from build123d import *

# Parameters (mm, degrees)
BOSS_EXTRUDE1_DEPTH = 8
SKETCH2_R           = 3.8805
CUT_EXTRUDE1_DEPTH  = 10
SKETCH5_W           = 15
SKETCH5_H           = 85
SKETCH5_R           = 2.5
SKETCH5_W_2         = 25
SKETCH5_H_2         = 105
SKETCH5_W_3         = 30
CUT_EXTRUDE4_DEPTH  = 1
CUT_EXTRUDE7_START  = 91
SKETCH10_R          = 2.5
CUT_EXTRUDE7_DEPTH  = 91
SKETCH12_W          = 165
SKETCH12_H          = 10
SKETCH12_R          = 2
CUT_EXTRUDE11_DEPTH = 3
SKETCH14_R          = 2.5
CUT_EXTRUDE14_DEPTH = 22


with BuildPart() as part:
    # Sketch1 → Boss-Extrude1 (new body)
    with BuildSketch(Plane.XY):
        Polygon((307.812229203, 127.5), (127.5, 307.812229203), (-127.5, 307.812229203), (-307.812229203, 127.5), (-307.812229203, -127.5), (-127.5, -307.812229203), (127.5, -307.812229203), (307.812229203, -127.5), align=None)
    extrude(amount=BOSS_EXTRUDE1_DEPTH)

    # Sketch2 → Cut-Extrude1 (cut)
    with BuildSketch(Plane.XY.offset(8)):
        with Locations((0, 200)):
            Circle(SKETCH2_R)
        with Locations((0, -200)):
            Circle(SKETCH2_R)
        Polygon((212.5, 105), (212.5, -105), (267.5, -105), (267.5, -40), (268.5, -40), (268.5, 0), (268.5, 40), (267.5, 40), (267.5, 105), align=None)
        Polygon((-267.5, 105), (-212.5, 105), (-212.5, -105), (-267.5, -105), (-267.5, -40), (-268.5, -40), (-268.5, 0), (-268.5, 40), (-267.5, 40), align=None)
    extrude(amount=-CUT_EXTRUDE1_DEPTH, mode=Mode.SUBTRACT)

    # Sketch5 → Cut-Extrude4 (cut)
    # profile 1 of 6: a face of its own
    with BuildSketch(Plane.XY.offset(8)):
        with Locations((80.5, 2.5)):
            Rectangle(SKETCH5_W, SKETCH5_H)
        with Locations(Location((78, 32.5, 0), (0, 0, 180))):
            Circle(SKETCH5_R, mode=Mode.SUBTRACT)
        with Locations(Location((78, -32.5, 0), (0, 0, 180))):
            Circle(SKETCH5_R, mode=Mode.SUBTRACT)
    # profile 2 of 6: a face of its own
    with BuildSketch(Plane.XY.offset(8)):
        with Locations((-185.5, 2.5)):
            Rectangle(SKETCH5_W_2, SKETCH5_H_2)
        with Locations((-183, -40)):
            Circle(SKETCH5_R, mode=Mode.SUBTRACT)
        with Locations((-183, 40)):
            Circle(SKETCH5_R, mode=Mode.SUBTRACT)
    # profile 3 of 6: a face of its own
    with BuildSketch(Plane.XY.offset(8)):
        with Locations((-133, 2.5)):
            Rectangle(SKETCH5_W_3, SKETCH5_H_2)
        with Locations((-133, -40)):
            Circle(SKETCH5_R, mode=Mode.SUBTRACT)
        with Locations((-133, 40)):
            Circle(SKETCH5_R, mode=Mode.SUBTRACT)
    # profile 4 of 6: a face of its own
    with BuildSketch(Plane.XY.offset(8)):
        with Locations((-80.5, 2.5)):
            Rectangle(SKETCH5_W, SKETCH5_H)
        with Locations((-78, -32.5)):
            Circle(SKETCH5_R, mode=Mode.SUBTRACT)
        with Locations((-78, 32.5)):
            Circle(SKETCH5_R, mode=Mode.SUBTRACT)
    # profile 5 of 6: a face of its own
    with BuildSketch(Plane.XY.offset(8)):
        with Locations((133, 2.5)):
            Rectangle(SKETCH5_W_3, SKETCH5_H_2)
        with Locations(Location((133, 40, 0), (0, 0, 180))):
            Circle(SKETCH5_R, mode=Mode.SUBTRACT)
        with Locations(Location((133, -40, 0), (0, 0, 180))):
            Circle(SKETCH5_R, mode=Mode.SUBTRACT)
    # profile 6 of 6: a face of its own
    with BuildSketch(Plane.XY.offset(8)):
        with Locations((185.5, 2.5)):
            Rectangle(SKETCH5_W_2, SKETCH5_H_2)
        with Locations(Location((183, 40, 0), (0, 0, 180))):
            Circle(SKETCH5_R, mode=Mode.SUBTRACT)
        with Locations(Location((183, -40, 0), (0, 0, 180))):
            Circle(SKETCH5_R, mode=Mode.SUBTRACT)
    extrude(amount=-CUT_EXTRUDE4_DEPTH, mode=Mode.SUBTRACT)

    # Sketch10 → Cut-Extrude7 (cut)
    with BuildSketch(Plane.XY.offset(CUT_EXTRUDE7_START)):
        with Locations(Location((-183, -40, 0), (0, 0, 180))):
            Circle(SKETCH10_R)
        with Locations(Location((-183, 40, 0), (0, 0, 180))):
            Circle(SKETCH10_R)
        with Locations((-133, -40)):
            Circle(SKETCH10_R)
        with Locations((-133, 40)):
            Circle(SKETCH10_R)
        with Locations(Location((-78, -32.5, 0), (0, 0, 180))):
            Circle(SKETCH10_R)
        with Locations(Location((-78, 32.5, 0), (0, 0, 180))):
            Circle(SKETCH10_R)
        with Locations(Location((78, 32.5, 0), (0, 0, 180))):
            Circle(SKETCH10_R)
        with Locations(Location((78, -32.5, 0), (0, 0, 180))):
            Circle(SKETCH10_R)
        with Locations(Location((133, 40, 0), (0, 0, 180))):
            Circle(SKETCH10_R)
        with Locations(Location((133, -40, 0), (0, 0, 180))):
            Circle(SKETCH10_R)
        with Locations(Location((183, 40, 0), (0, 0, 180))):
            Circle(SKETCH10_R)
        with Locations(Location((183, -40, 0), (0, 0, 180))):
            Circle(SKETCH10_R)
    extrude(amount=-CUT_EXTRUDE7_DEPTH, mode=Mode.SUBTRACT)

    # Sketch12 → Cut-Extrude11 (cut)
    with BuildSketch(Plane.XY.offset(8)):
        with Locations((0, 252.812229203)):
            Rectangle(SKETCH12_W, SKETCH12_H)
        with Locations((-72.5, 252.812229203)):
            Circle(SKETCH12_R, mode=Mode.SUBTRACT)
        with Locations(Location((72.5, 252.812229203, 0), (0, 0, 180))):
            Circle(SKETCH12_R, mode=Mode.SUBTRACT)
    extrude(amount=-CUT_EXTRUDE11_DEPTH, mode=Mode.SUBTRACT)

    # Sketch14 → Cut-Extrude14 (cut)
    with BuildSketch(Plane.XY):
        with Locations((-72.5, 252.812229203)):
            Circle(SKETCH14_R)
        with Locations(Location((72.5, 252.812229203, 0), (0, 0, 180))):
            Circle(SKETCH14_R)
    extrude(amount=CUT_EXTRUDE14_DEPTH, mode=Mode.SUBTRACT)


solid = part.part
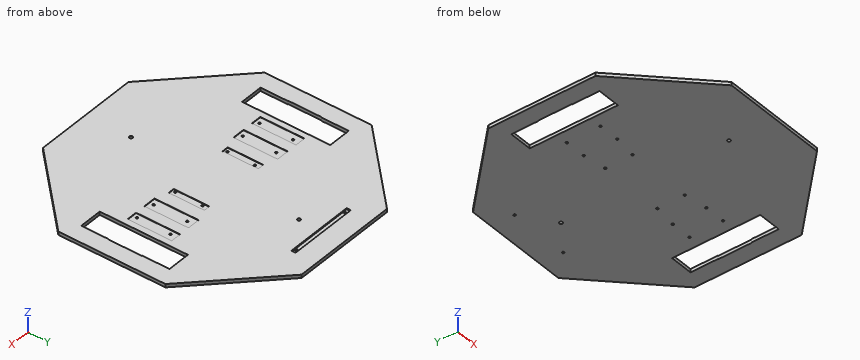
The listing builds one solid part. Answer for the finished solid, in the listing's coordinates (mm). Give positions to 0.01 mm unless a question says otherwise; leave off trailing zeros. Loops run counter-clockwise (first coordinate to the right, second up) from the corner with the lowest first, then second, coordinate; pieces in that order, holes last. Notation, with made-up numbers: (88.25, 40.5) - (143.25, 40.5) arc R10 cw to (143.25, 58.5) - close; hole circle Ø4 at (45.25, -7.5). An arc over 180 degrees is marked (long way). Write each question's results on one line, items separated by ' | '.
1. Consider probe 1 along X at (y, z) = (5.5, 3.5); probe 2 along Y at (x, z) = (78, 4); probe 3 along Y at (x, z) = (134.5, 3). Determine where each line is inside the solid, lowest interval first. Write a range as from..to.
Resolved:
probe 1: x = -307.81..-268.5, -212.5..212.5, 268.5..307.81 | probe 2: y = -307.81..-35, -30..30, 35..307.81 | probe 3: y = -300.81..-42, -38..38, 42..300.81
2. Find section C-C, the plane z = 2. Count the separate pieces of the cut face and the enclosed holes in it, then the cut area to 3 significant figures.
Resolved:
separate pieces: 1 | enclosed holes: 18 | area: 290,000 mm^2
3. Flat-ended cylindrical pins translate along their axes: P1, Ø6.5, axis at x = -72.5, y = 252.81, coming from the +Z side; P2, Ø1.1, axis at x = -268, z = 2.5, coming from the -Y side; P3, Ø8, axis at x = -183, y = -40, coming from the -Z side; P4, Ø0.8, axis at x = -190.5, z = 7.5, coming from the -Y side. Find the tip coordinate at first contact, or state that the pin passes through.
Resolved:
P1: stops at z = 5 | P2: stops at y = -167.86 | P3: stops at z = 0 | P4: stops at y = -245.21
4. Find section A-A, the plane x = -223.5. Write down the section's boundary in (y, z).
Resolved:
outline: (-211.81, 0) - (-105, 0) - (-105, 8) - (-211.81, 8) - close; (105, 0) - (211.81, 0) - (211.81, 8) - (105, 8) - close
5. Find section B-B, the plane y = -149.5. Write down the section's boundary in (x, z).
Resolved:
outline: (-285.81, 0) - (285.81, 0) - (285.81, 8) - (-285.81, 8) - close
